```python
from build123d import *

# Parameters (mm, degrees)
SKETCH1_W                = 76.2
SKETCH1_H                = 50.8
SKETCH1_R                = 1.5875
BOSS_EXTRUDE1_DEPTH      = 2.54
SKETCH2_R                = 3.175
BOSS_EXTRUDE2_DEPTH      = 5.08
BOSS_EXTRUDE2_DEPTH_BACK = 2.54


with BuildPart() as part:
    # Sketch1 → Boss-Extrude1 (new body)
    with BuildSketch(Plane.XY):
        Rectangle(SKETCH1_W, SKETCH1_H)
        with Locations((-34.29, 22.225)):
            Circle(SKETCH1_R, mode=Mode.SUBTRACT)
        with Locations((34.29, 22.225)):
            Circle(SKETCH1_R, mode=Mode.SUBTRACT)
        with Locations((34.29, -22.225)):
            Circle(SKETCH1_R, mode=Mode.SUBTRACT)
        with Locations((-34.29, -22.225)):
            Circle(SKETCH1_R, mode=Mode.SUBTRACT)
    extrude(amount=BOSS_EXTRUDE1_DEPTH)

    # Sketch2 → Boss-Extrude2 (add, two sides)
    with BuildSketch(Plane.XY.offset(2.54)) as boss_extrude2_sk:
        with Locations((-25.4, 24.13)):
            Circle(SKETCH2_R)
        with Locations((-26.67, -24.13)):
            Circle(SKETCH2_R)
        with Locations((25.4, 8.89)):
            Circle(SKETCH2_R)
        with Locations((25.4, -19.05)):
            Circle(SKETCH2_R)
    extrude(amount=BOSS_EXTRUDE2_DEPTH)
    extrude(boss_extrude2_sk.sketch, amount=-BOSS_EXTRUDE2_DEPTH_BACK)


solid = part.part
```
Design review of the part built by this model. Coordinates are the model's own, in mm. A direction names the side the tool comes from. Coordinates: 2 decimals unless noted, no trailing zeros. Write each loop counter-clockwise with the first axis right and the second up, starting at its lowest first coordinate (ties: lowest second). Pieces come first, ordered by that corner, then holes.
1) Add section C-C (z = 1.5). State how many separate pieces and enclosed holes the cut face has, plus the area to 3 significant figures.
2) Add section A-A (x = -34.29). Write out the cut boundary in (y, z), plus the area to 3 significant figures.
3) Machinability: for faces 4 (the flat face through (7, 25.4, 1)), 5 (the flat face through (-34, -25.4, 1)), 6 (the cylindrical face through (28.43, -18.1, 5.04)), 7 (the flat face through (-33, 25.4, 1)), 8 (the flat face through (7, -25.4, 1)), which of the approach directions +Z, -Z, +X, -X, +Y, -Y give a long, thin tool a straight path to every point of the face, cutting with its end or side? Answer none if there is none.
4) Insertion check: pin 1 (2 mm diameter, centred on x = -15.5, z = 3.5, fed in from +Y); pin 2 (2 mm diameter, centred on x = 8, y = -9.5, fed in from +Z); pin 3 (3 mm diameter, centred on x = 0.5, z = 1, fed in from -Y); pin 4 (1.5 mm diameter, centred on x = -2.5, z = 4, fed in from -Y). Each pin has a flat end and moves straight along its axis. Give the tip position at first contact, or say it passes through.
5) Add section B-B (z = 6.5). Write out the cut boundary in (x, y) (3 decimals), plus the area to 3 significant figures.
6) Mouldability with a two-part tool opening along X and no side actions: class faces 1 (the flat face through (38.1, 0, 1)), 2 (the cylindrical face through (35.143, -20.886, 1.252)), 3 (the flat face through (25, 9, 7.62)) as +X half, -X half, draft (parallel to the pull), parting line (faces both ways), or undercut.
7) Add section D-D (y = -19.05). Write out the cut boundary in (x, z) (3 decimals), plus the area to 3 significant figures.
8) To check wall thickness, follow L1, parallel to Y at x = 34.29, z = 2; L2, parallel to X at y = 22, z = 1.5; L3, parallel to Z at x = 17, y = 12.5. State the ranges of each line that lie inside material, in increasing order.
Check result:
1. separate pieces: 1
1. enclosed holes: 4
1. area: 3,860 mm2
2. outline: (-25.4, 0) - (-23.81, 0) - (-23.81, 2.54) - (-25.4, 2.54) - close; (-20.64, 0) - (20.64, 0) - (20.64, 2.54) - (-20.64, 2.54) - close; (23.81, 0) - (25.4, 0) - (25.4, 2.54) - (23.81, 2.54) - close
2. area: 113 mm2
3. face 4: +Z, -Z, +X, +Y
3. face 5: +Z, -Z, -X, -Y
3. face 6: +Z
3. face 7: +Z, -Z, -X, +Y
3. face 8: +Z, -Z, +X, -Y
4. pin 1: stops at y = 25.4
4. pin 2: stops at z = 2.54
4. pin 3: stops at y = -25.4
4. pin 4: passes through
5. outline: circle Ø6.35 at (-26.67, -24.13); circle Ø6.35 at (-25.4, 24.13); circle Ø6.35 at (25.4, -19.05); circle Ø6.35 at (25.4, 8.89)
5. area: 127 mm2
6. face 1: +X half
6. face 2: undercut
6. face 3: draft
7. outline: (-38.1, 0) - (38.1, 0) - (38.1, 2.54) - (28.575, 2.54) - (28.575, 7.62) - (22.225, 7.62) - (22.225, 2.54) - (-38.1, 2.54) - close
7. area: 226 mm2
8. L1: y = -25.4 to -23.81, -20.64 to 20.64, 23.81 to 25.4
8. L2: x = -38.1 to -35.86, -32.72 to 32.72, 35.86 to 38.1
8. L3: z = 0 to 2.54
